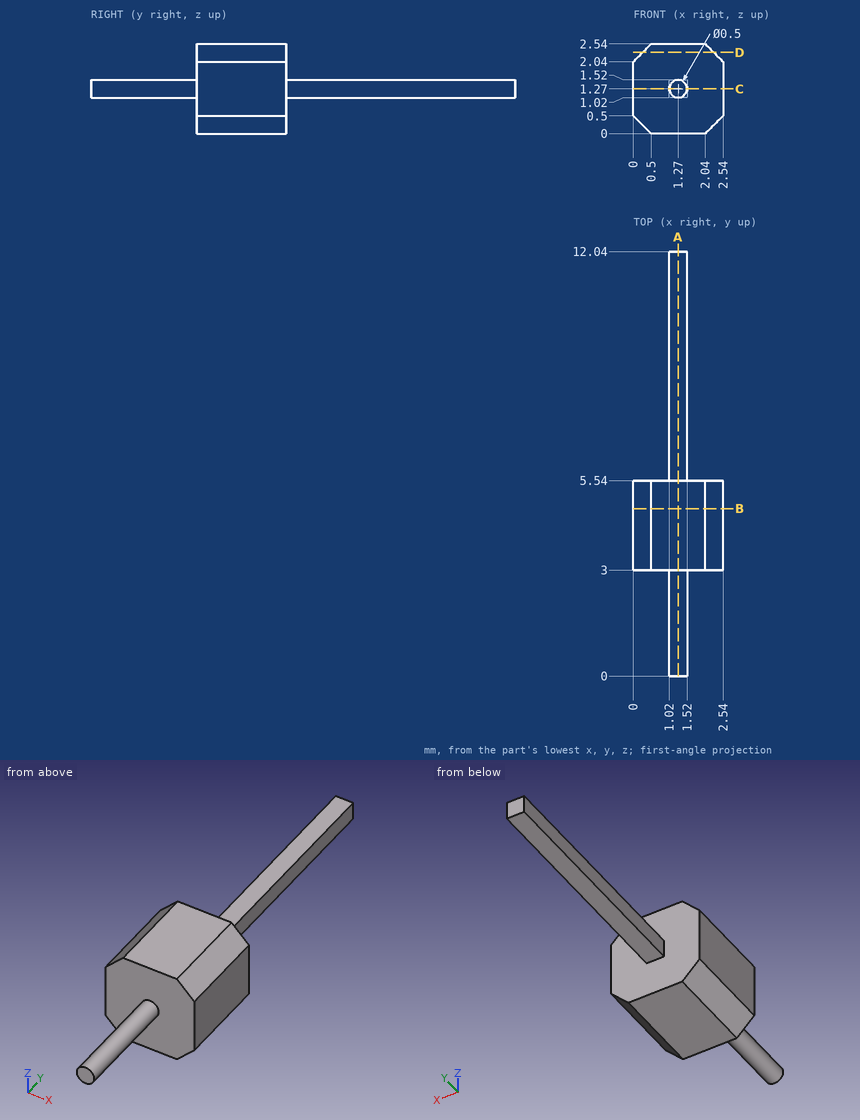
Geometry: see drawing. Coordinates: mm, zero at the bounding-box minimum. Give positions to 0.01 mm unless a question says otherwise; leave off trailing zeros. Order: outer loops, then holes, each group sorted by start corner. A loop starts at its lowest first (then second) coordinate and runs counter-clockwise, first axis right, second up. Notation, with made-up numbers: (60, 18.5) -> (73, 18.5) arc R15 ccw to (73, 26.5) -> close; hole circle Ø10 at (-24.5, -6.75). An arc over 180 degrees is marked (long way). Write each question's results on one line, items separated by ' | '. Start each with the question number.
1) Section D-D (z = 2.3). Return loops of the section in (x, y), then the cut area to 3 significant figures.
2) Section B-B (y = 4.75). Return loops of the section in (x, z).
3) Section A-A (x = 1.27). Return loops of the section in (y, z).
4) First-contact query: pin 1 (0.6 mm diameter, centred on y = 8, z = 1, fed in from +X). Flat tip, straight axial feed; report the tip coordinate or a pass-through.
5) Section C-C (z = 1.27). Return loops of the section in (x, y).
6) Line query: line 1 (Y direction, x = 0.7, z = 2); line 2 (Z direction, x = 1.4, y = 9.25). Output: solid intervals per line, ascending. Write a range as from..to.
Calculated:
1) outline: (0.26, 3) -> (2.28, 3) -> (2.28, 5.54) -> (0.26, 5.54) -> close | area: 5.13 mm2
2) outline: (0, 0.5) -> (0.5, 0) -> (2.04, 0) -> (2.54, 0.5) -> (2.54, 2.04) -> (2.04, 2.54) -> (0.5, 2.54) -> (0, 2.04) -> close
3) outline: (0, 1.02) -> (3, 1.02) -> (3, 0) -> (5.54, 0) -> (5.54, 1.02) -> (12.04, 1.02) -> (12.04, 1.52) -> (5.54, 1.52) -> (5.54, 2.54) -> (3, 2.54) -> (3, 1.52) -> (0, 1.52) -> close
4) pin 1: x = 1.52
5) outline: (0, 3) -> (1.02, 3) -> (1.02, 0) -> (1.52, 0) -> (1.52, 3) -> (2.54, 3) -> (2.54, 5.54) -> (1.52, 5.54) -> (1.52, 12.04) -> (1.02, 12.04) -> (1.02, 5.54) -> (0, 5.54) -> close
6) line 1: 3..5.54 | line 2: 1.02..1.52
